The listing builds one solid part. Answer for the finished solid, in the listing's coordinates (mm). Face numbers are marked on the shaded views. Coordinates: 2 decimals unless noted, no trailing zeros. Loops run counter-clockwise (first coordinate to the right, second up) from the corner with the lowest first, then second, coordinate; pieces in that order, holes last. Notation, with made-up numbers: M 47.5,41 L 106.5,41 A24 cw 106.5,80 Z; hole C 36.5,-32 d2. An arc over 180 degrees is marked long. Answer in a Markdown table with one row per item. Add a question column.
from build123d import *

# Parameters (mm, degrees)
SKETCH1_W           = 30.988
SKETCH1_H           = 30.988
SKETCH1_R           = 5.7277
BOSS_EXTRUDE1_DEPTH = 3.175
SKETCH2_R           = 10.8712
CUT_EXTRUDE2_DEPTH  = 3.2512


with BuildPart() as part:
    # Sketch1 → Boss-Extrude1 (new body)
    with BuildSketch(Plane.XY):
        with Locations((15.494, 15.494)):
            Rectangle(SKETCH1_W, SKETCH1_H)
        with Locations((15.494, 15.494)):
            Circle(SKETCH1_R, mode=Mode.SUBTRACT)
    extrude(amount=BOSS_EXTRUDE1_DEPTH)

    # Sketch2 → Cut-Extrude2 (cut)
    with BuildSketch(Plane(origin=(0, 0, 0), x_dir=(-1, 0, 0), z_dir=(0, 0, -1))):
        with Locations((-15.494, 15.494)):
            Circle(SKETCH2_R)
    extrude(amount=-CUT_EXTRUDE2_DEPTH, mode=Mode.SUBTRACT)


solid = part.part
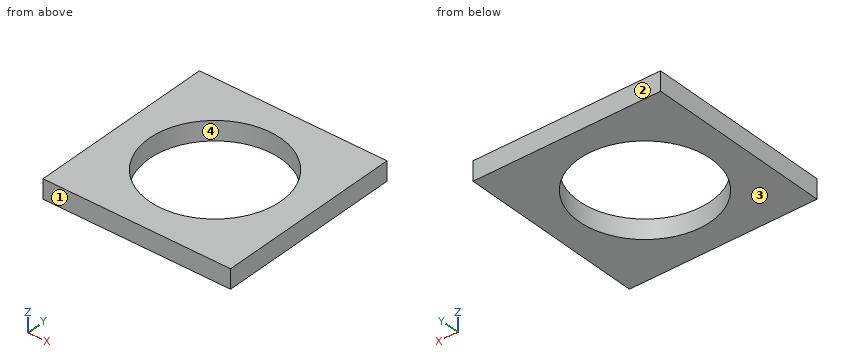
(1) The mould has two halves that part along Y. Classify the marked faces 1, 2, 3 and 4: released by +Y, released by -Y, zero draft, split by the parting line, or undercut.
(2) A cutting plane is placed at A-A (x = 15.5). Give the vertices of the cut face in (y, z) (3 decimals).
(3) Straight lines are drawn through the part: line 1 (X direction, y = 7, z = 2.3); line 2 (X direction, y = 7.5, z = 1.55); line 3 (Y direction, x = 14, z = 0.25). For each, find the intervals that lie inside material, in ascending order.
(4) A cutting plane is placed at B-B (y = 26). Give the vertices of the cut face in (x, z) (3 decimals).
(5) A cutting plane is placed at C-C (z = 0.9). Give the vertices of the cut face in (x, y), plus the area to 3 significant figures.
Solved:
| question | item | result |
|---|---|---|
| 1 | face 1 | released by -Y |
| 1 | face 2 | released by +Y |
| 1 | face 3 | zero draft |
| 1 | face 4 | undercut |
| 2 | outline | M 0,0 L 4.623,0 L 4.623,3.175 L 0,3.175 Z; M 26.365,0 L 30.988,0 L 30.988,3.175 L 26.365,3.175 Z |
| 3 | line 1 | x = 0 to 8.71, 22.28 to 30.99 |
| 3 | line 2 | x = 0 to 8.13, 22.86 to 30.99 |
| 3 | line 3 | y = 0 to 4.73, 26.26 to 30.99 |
| 4 | outline | M 0,0 L 12.7,0 L 12.7,3.175 L 0,3.175 Z; M 18.288,0 L 30.988,0 L 30.988,3.175 L 18.288,3.175 Z |
| 5 | outline | M 0,0 L 30.99,0 L 30.99,30.99 L 0,30.99 Z; hole C 15.49,15.49 d21.74 |
| 5 | area | 589 mm² |
